Job drawing, mm, ordinate dimensions from the low corner. One solid piece. A direction names the side the tool comes from. Give positions to 0.01 mm unless a question says otherwise; leave off trailing zeros. Order: outer loops, then holes, each group sorted by start corner. A loop starts at its lowest first (then second) coordinate and runs counter-clockwise, first axis right, second up.
Item 1: Band-saw the part on B-B on x = 25.5. Give the cut face in (y, z).
Item 2: Band-saw the part on A-A on y = 14. Count the separate pieces of the cut face and the enclosed holes in it, plus the area to 3 significant figures.
Item 3: Which spindle directions (+Z, -Z, +X, -X, +Y, -Y) get a long thin tool onto all of the face, cutting with end or side? Do the marked faces 5 and 6. Say none if no direction does.
Item 4: Two-plate mould, pull along X, no slides. Class the marked faces 1, 2, 3 and 4: released by +X, released by -X, zero draft, split by the parting line, or undercut.
Item 5: Band-saw the part on C-C on y = 21.25. Give the cut face in (x, z).
Item 6: Band-saw the part on D-D on z = 14.5. Give the cut face in (x, y).
Item 7: Flat gauge pins, fed straight in: P1, Ø2.5, axis at x = 49, y = 16, coming from the -Z side; P2, Ø0.9, axis at x = 1.5, y = 16.5, coming from the +Z side; P3, Ø1.4, axis at x = 50, y = 11, coming from the +Z side; P4, Ø0.9, axis at x = 49.5, z = 25.5, coming from the -Y side. Where does each tip first touch, or does it go through?
Item 8: Wall check: L1, parallel to X at y = 3.5, z = 34; L2, parallel to Y at x = 25.5, z = 0.75; L3, parallel to Z at x = 16.5, y = 15.5. Give the ranges that are in metal, low to high.
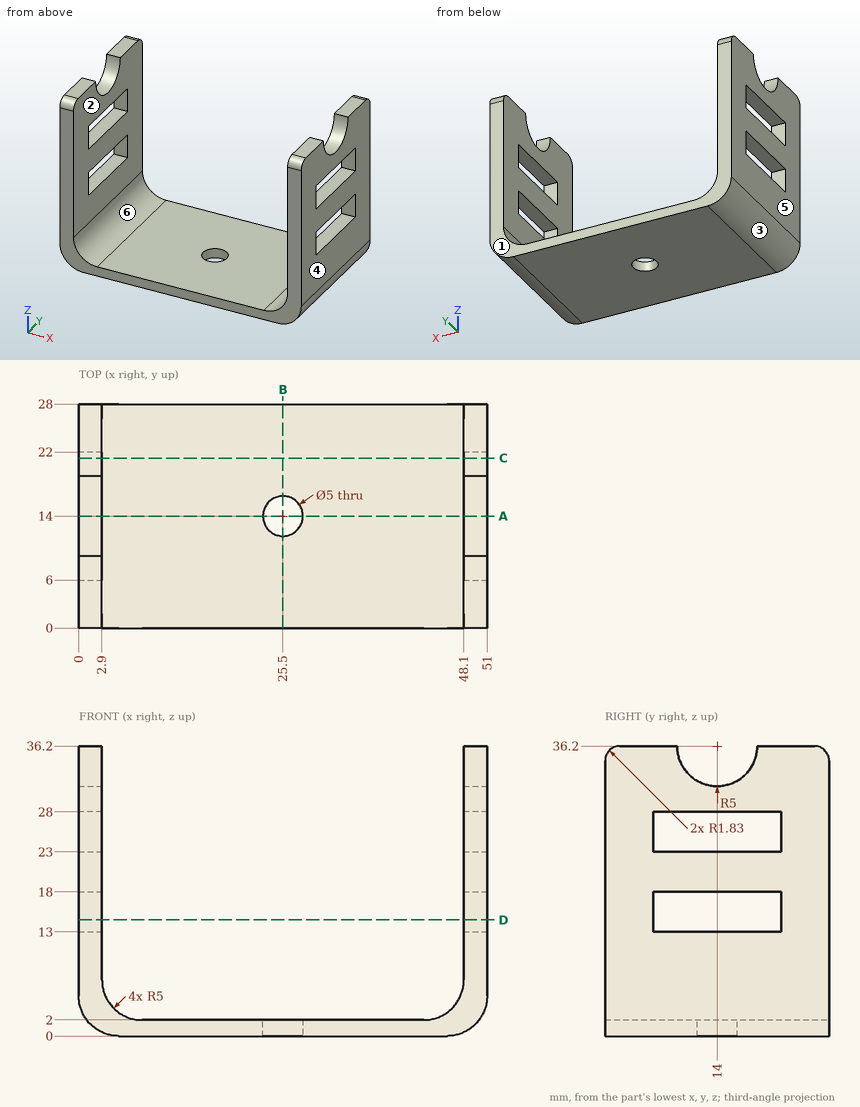
The answers:
1. outline: (0, 0) - (11.5, 0) - (11.5, 2) - (0, 2) - close; (16.5, 0) - (28, 0) - (28, 2) - (16.5, 2) - close
2. separate pieces: 6
2. enclosed holes: 0
2. area: 203 mm2
3. face 5: +Z, -Z, -X, +Y, -Y
3. face 6: +Z, +Y, -Y
4. face 1: zero draft
4. face 2: undercut
4. face 3: released by -X
4. face 4: released by +X
5. outline: (0, 5) arc R5 ccw to (5, 0) - (46, 0) arc R5 ccw to (51, 5) - (51, 13) - (48.1, 13) - (48.1, 7) arc R5 cw to (43.1, 2) - (7.9, 2) arc R5 cw to (2.9, 7) - (2.9, 13) - (0, 13) - close; (0, 18) - (2.9, 18) - (2.9, 23) - (0, 23) - close; (0, 28) - (2.9, 28) - (2.9, 36.2) - (0, 36.2) - close; (48.1, 18) - (51, 18) - (51, 23) - (48.1, 23) - close; (48.1, 28) - (51, 28) - (51, 36.2) - (48.1, 36.2) - close
6. outline: (0, 0) - (2.9, 0) - (2.9, 6) - (0, 6) - close; (0, 22) - (2.9, 22) - (2.9, 28) - (0, 28) - close; (48.1, 0) - (51, 0) - (51, 6) - (48.1, 6) - close; (48.1, 22) - (51, 22) - (51, 28) - (48.1, 28) - close
7. P1: stops at z = 0.32
7. P2: stops at z = 32.16
7. P3: stops at z = 32.84
7. P4: stops at y = 0
8. L1: x = 0 to 2.9, 48.1 to 51
8. L2: y = 0 to 11.5, 16.5 to 28
8. L3: z = 0 to 2
